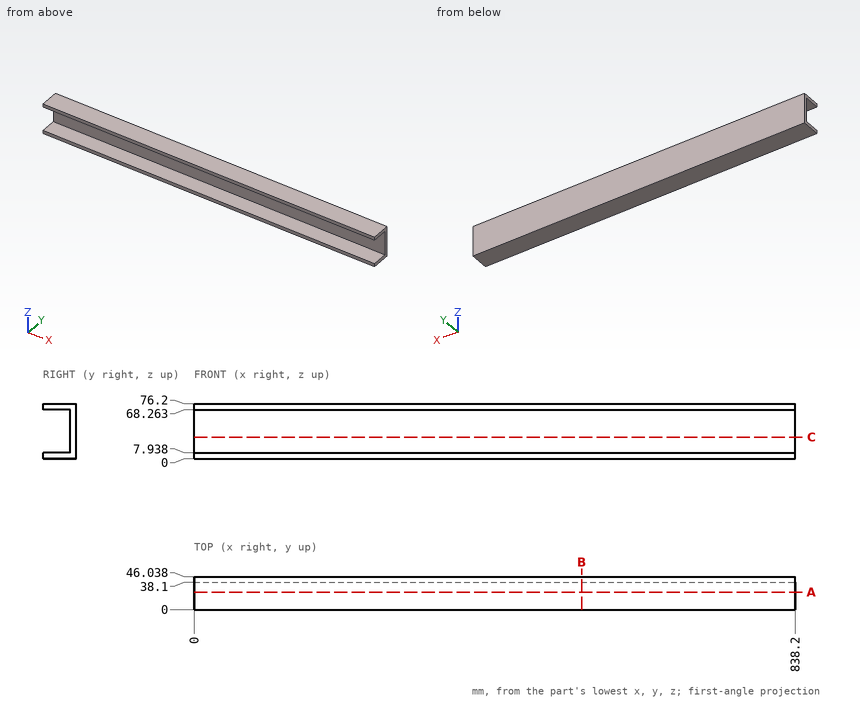
The figure shows three views and two pictorial views of one solid part (mm, origin at its lowest corner). Answer the questions. Coordinates: 2 decimals unless noted, no trailing zeros. Write each loop counter-clockwise with the first axis right and the second up, starting at its lowest first coordinate (ties: lowest second). Pieces come first, ordered by that corner, then holes. Notation, with made-up numbers: (48.5, 13.25) -> (105.5, 13.25) arc R4 cw to (105.5, 17.25) -> close; hole circle Ø11 at (23, 5). An arc over 180 degrees is marked (long way). Return JSON: item names as keys, results as strings.
1. A cutting plane is placed at B-B (x = 540.5). Determine the outline of the cut face in (y, z), and give its area (3 significant figures).
Found:
{"outline": "(0, 0) -> (46.04, 0) -> (46.04, 76.2) -> (0, 76.2) -> (0, 68.26) -> (38.1, 68.26) -> (38.1, 7.94) -> (0, 7.94) -> close", "area": "1,210 mm2"}
2. Find the intervals of material crossed by line 1 along Z through (x, y) = (602, 22.5); line 2 along Y through (x, z) = (717.5, 47), in increasing order. Write a range as from..to.
Found:
{"line 1": "0..7.94, 68.26..76.2", "line 2": "38.1..46.04"}
3. A cutting plane is placed at C-C (z = 30). Determine the outline of the cut face in (x, y), and give its area (3 significant figures).
Found:
{"outline": "(0, 38.1) -> (838.2, 38.1) -> (838.2, 46.04) -> (0, 46.04) -> close", "area": "6,650 mm2"}
4. A cutting plane is placed at A-A (y = 24.5). Determine the outline of the cut face in (x, z), and give its area (3 significant figures).
Found:
{"outline": "(0, 0) -> (838.2, 0) -> (838.2, 7.94) -> (0, 7.94) -> close; (0, 68.26) -> (838.2, 68.26) -> (838.2, 76.2) -> (0, 76.2) -> close", "area": "13,300 mm2"}
